```python
from build123d import *

# Parameters (mm, degrees)
SKETCH_1_W          = 20
SKETCH_1_H          = 20
SKETCH_1_W_2        = 18
SKETCH_1_H_2        = 18
EXTRUDE_1_DEPTH     = 140
SKETCH_2_W          = 20
SKETCH_2_H          = 20
EXTRUDE_2_DEPTH     = 20
SKETCH_3_R          = 3
CUT_EXTRUDE_1_DEPTH = 2


with BuildPart() as part:
    # 草图1 → 凸台-拉伸1 (new body)
    with BuildSketch(Plane(origin=(0, 0, 0), x_dir=(1, 0, 0), z_dir=(0, 1, 0))):
        Rectangle(SKETCH_1_W, SKETCH_1_H)
        Rectangle(SKETCH_1_W_2, SKETCH_1_H_2, mode=Mode.SUBTRACT)
    extrude(amount=EXTRUDE_1_DEPTH)

    # 草图2 → 凸台-拉伸2 (add)
    with BuildSketch(Plane.XZ):
        Rectangle(SKETCH_2_W, SKETCH_2_H)
    extrude(amount=EXTRUDE_2_DEPTH)

    # 草图3 → 切除-拉伸1 (cut)
    with BuildSketch(Plane.XY.offset(10)):
        with Locations((0, 120)):
            Circle(SKETCH_3_R)
    extrude(amount=-CUT_EXTRUDE_1_DEPTH, mode=Mode.SUBTRACT)


solid = part.part
```
Check sheet for the modelled part. Datum: model origin and axes. Units: mm. A direction names the side the tool comes from. Coordinates: 2 decimals unless noted, no trailing zeros. Order: outer loops, then holes, each group sorted by start corner. A loop starts at its lowest first (then second) coordinate and runs counter-clockwise, first axis right, second up. Notation, with made-up numbers: M 37.5,56.5 L 72.5,56.5 A30 cw 72.5,79.5 Z; hole C -29,20.5 d10. An arc over 180 degrees is marked long. One line per question, with ' | ' between items. Start each with the question number.
Item 1: Sectioned sample at B-B on z = 0.75. Record the cut outline in (x, y), and give its area (3 significant figures).
Item 2: Material ranges on line 1 (Y direction, x = 0, z = 9.6); line 2 (X direction, y = 56, z = -8.25), recorded low to high.
Item 3: Sectioned sample at A-A on x = 0. Record the cut outline in (y, z), and give its area (3 significant figures).
Item 4: Mould release check, pull along Z, two halves, no side actions. Record for faces 1 (the flat face through (9, 69, 0)), 2 (the flat face through (-0.8, 140, 9.6)), 3 (the flat face through (0, 69, -9)), 4 (the flat face through (0, 61, 10)): pulls with the +Z half, pulls with the -Z half, needs draft (parallel to the pull), parting line crosses it, or undercut.
Item 5: Sectioned sample at C-C on y = 107. Record the cut outline in (x, z), and give its area (3 significant figures).
Item 6: Access from +Z, -Z, +X, -X, +Y, -Y to the whole of each face (thin tool, end or side, straight path). Record for faces 5 (the cylindrical face through (-0.391, 122.974, 9.507)), 6 (the flat face through (0, 69, 9)), 7 (the flat face through (10, 61, 0)).
Answer below:
1) outline: M -10,-20 L 10,-20 L 10,140 L 9,140 L 9,0 L -9,0 L -9,140 L -10,140 Z | area: 680 mm^2
2) line 1: y = -20 to 117, 123 to 140 | line 2: x = -10 to -9, 9 to 10
3) outline: M -20,-10 L 140,-10 L 140,-9 L 0,-9 L 0,9 L 117,9 L 117,10 L -20,10 Z; M 123,9 L 140,9 L 140,10 L 123,10 Z | area: 674 mm^2
4) face 1: undercut | face 2: needs draft | face 3: undercut | face 4: pulls with the +Z half
5) outline: M -10,-10 L 10,-10 L 10,10 L -10,10 Z; hole M -9,-9 L 9,-9 L 9,9 L -9,9 Z | area: 76.0 mm^2
6) face 5: +Z | face 6: +Y | face 7: +Z, -Z, +X, +Y, -Y
